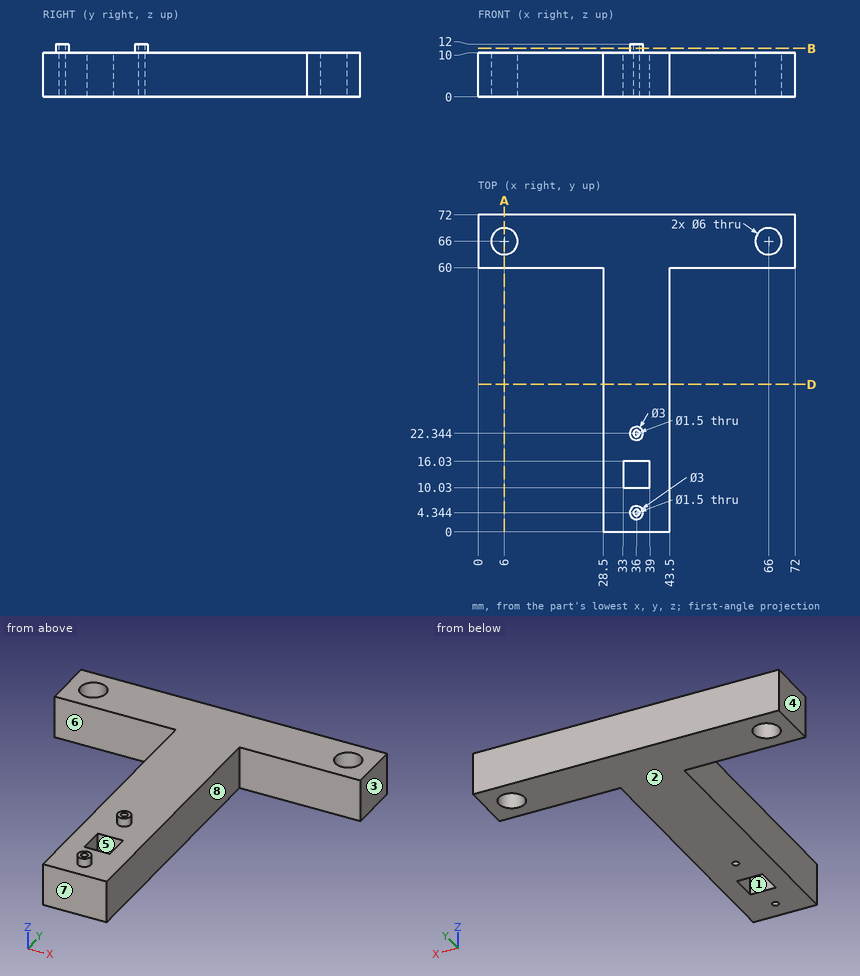
Check sheet for the drawn part. Datum: minimum x, y, z corner. Units: mm. A direction names the side the tool comes from. Round coordinates to 2 decimals unless told otherwise and drop trailing zeros. Order: outer loops, then holes, each group sorted by start corner. A loop starts at its lowest first (then second) coordinate and runs counter-clockwise, first axis right, second up.
1. Access from +Z, -Z, +X, -X, +Y, -Y to the whole of each face (thin tool, end or side, straight path). Record for the marked faces 4, 5, 6, 7 and 8.
Final values:
face 4: +Z, -Z, -X, +Y, -Y
face 5: +Z, -Z
face 6: +Z, -Z, -X, -Y
face 7: +Z, -Z, +X, -X, -Y
face 8: +Z, -Z, +X, -Y
2. Section check B-B on z = 11. State how many separate pieces and enclosed holes the cut face has, then the cut area to 3 significant figures.
Final values:
separate pieces: 2
enclosed holes: 2
area: 10.6 mm2
3. Thickness scan on L1, parallel to Y at x = 36, z = 3.25 (1 decimal); L2, parallel to Y at x = 66, z = 4.25; L3, parallel to X at y = 12.5, z = 5. Record the ranges inside material, lowest first.
Final values:
L1: y = 0 to 3.6, 5.1 to 10, 16 to 21.6, 23.1 to 72
L2: y = 60 to 63, 69 to 72
L3: x = 28.5 to 33, 39 to 43.5
4. Section check D-D on y = 33.5. Record the cut outline in (x, z), then the cut area to 3 significant figures.
Final values:
outline: (28.5, 0) - (43.5, 0) - (43.5, 10) - (28.5, 10) - close
area: 150 mm2
5. Section check A-A on x = 6. Record the cut outline in (y, z).
Final values:
outline: (60, 0) - (63, 0) - (63, 10) - (60, 10) - close; (69, 0) - (72, 0) - (72, 10) - (69, 10) - close
6. Go/stop test with flat-tipped pins: P1, Ø4, axis at x = 23.5, z = 4.5, coming from the -Y side; P2, Ø1, axis at x = 44.5, y = 62.5, coming from the +Z side; P3, Ø5, axis at y = 40.5, z = 5.5, coming from the +X side. Record where each tip stops, or that it passes through.
Final values:
P1: stops at y = 60
P2: stops at z = 10
P3: stops at x = 43.5
7. Release check for a two-part mould opening along X. For the marked faces 1, 2 and 3 record: +X half, -X half, draft (parallel to the pull), parting line (faces both ways), or undercut.
Final values:
face 1: undercut
face 2: draft
face 3: +X half
